Job drawing, mm, ordinate dimensions from the low corner. One solid piece. Give positions to 0.01 mm unless a question says otherwise; leave off trailing zeros. Write each loop counter-clockwise with the first axis right and the second up, starting at its lowest first coordinate (ties: lowest second). Pieces come first, ordered by that corner, then holes. Notation, with made-up numbers: (-33, 55.25) - (15, 55.25) arc R28 ccw to (15, 92.25) - close; hole circle Ø1 at (86, 81.25). An arc over 180 degrees is marked (long way). Answer in a Markdown table with one row per item. Add a question column.
1. Band-saw the part on C-C on x = 12.7. Write the cut outline in (y, z) (3 decimals), plus the area to 3 significant figures.
2. Band-saw the part on D-D on x = 55. Write the cut outline in (y, z) (3 decimals).
3. Band-saw the part on A-A on z = 91. Write the cut outline in (x, y) (3 decimals).
4. Probe line 1 along Z through (x, y) = (218.3, 6.25); line 2 along Z through (x, y) = (70.5, 6.25); line 3 along X through (y, z) = (4.25, 37.5). List the from-to ranges inside material, lowest first.
5. Drop a flat-ended pin along its axis: pin 1 Ø5 at (x, y) = (203.5, 4.5) entering from -Z. Give the stop position or say it passes through.
6. Band-saw the part on B-B on y = 7. Write the cut outline in (x, z).
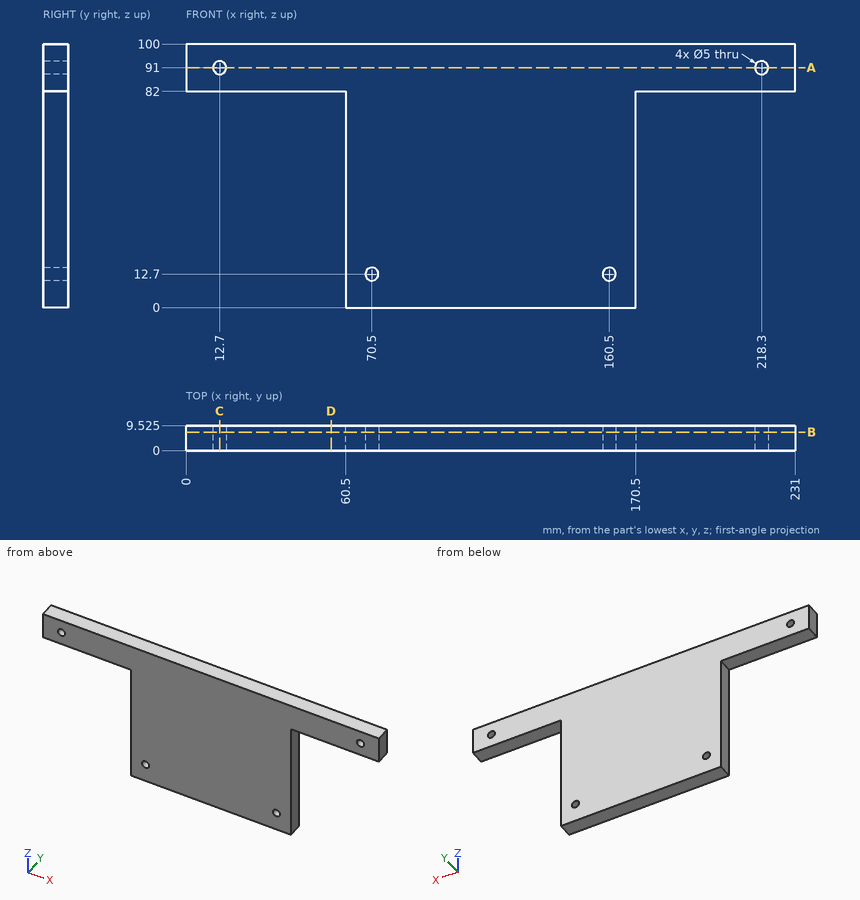
Values:
| question | item | result |
|---|---|---|
| 1 | outline | (0, 82) - (9.525, 82) - (9.525, 88.5) - (0, 88.5) - close; (0, 93.5) - (9.525, 93.5) - (9.525, 100) - (0, 100) - close |
| 1 | area | 124 mm² |
| 2 | outline | (0, 82) - (9.525, 82) - (9.525, 100) - (0, 100) - close |
| 3 | outline | (0, 0) - (10.2, 0) - (10.2, 9.525) - (0, 9.525) - close; (15.2, 0) - (215.8, 0) - (215.8, 9.525) - (15.2, 9.525) - close; (220.8, 0) - (231, 0) - (231, 9.525) - (220.8, 9.525) - close |
| 4 | line 1 | z = 82 to 88.5, 93.5 to 100 |
| 4 | line 2 | z = 0 to 10.2, 15.2 to 100 |
| 4 | line 3 | x = 60.5 to 170.5 |
| 5 | pin 1 | stops at z = 82 |
| 6 | outline | (0, 82) - (60.5, 82) - (60.5, 0) - (170.5, 0) - (170.5, 82) - (231, 82) - (231, 100) - (0, 100) - close; hole circle Ø5 at (12.7, 91); hole circle Ø5 at (70.5, 12.7); hole circle Ø5 at (160.5, 12.7); hole circle Ø5 at (218.3, 91) |
